Autodesk Inventor part; units mm, degrees
ref_plane "YZ Plane" through (0, 0, 0) normal (1, 0, 0) x (0, 1, 0)
ref_plane "XZ Plane" through (0, 0, 0) normal (0, 1, 0) x (-1, 0, 0)
ref_plane "XY Plane" through (0, 0, 0) normal (0, 0, 1) x (1, 0, 0)
sketch "Sketch1" plane through (0, 0, 0) normal (0, 1, 0) x (-1, 0, 0)
  line L0 (101.6, -38.1) -> (-101.6, -38.1)
  line L1 (-101.6, -38.1) -> (-101.6, 38.1)
  line L2 (-101.6, 38.1) -> (101.6, 38.1)
  line L3 (101.6, 38.1) -> (101.6, -38.1)
  line L4 (101.6, -38.1) -> (-101.6, 38.1) construction
  line L5 (-101.6, -38.1) -> (101.6, 38.1) construction
  point P0 (0, 0)
  dimension "d0" = 203.2
  dimension "d1" = 76.2
extrude "Extrusion1" add sketch "Sketch1" against normal blind 3.175
sketch "Sketch2" plane through (0, 0, 0) normal (0, 1, 0) x (1, 0, 0)
  line L0 (-101.6, 38.1) -> (101.6, 38.1) construction
  line L1 (0, 38.1) -> (0, -38.1) construction
  line L2 (101.6, -38.1) -> (-101.6, -38.1) construction
  point P0 (0, 0)
  point P1 (-63.5, 19.05)
  point P2 (0, 0)
  point P3 (63.5, 19.05)
  dimension "d4" = 19.05
  dimension "d5" = 63.5
hole "Hole1" at (-63.5, 0, -19.05) at (63.5, 0, -19.05) direction (0, -1, 0) diameter 22.225 end through all
fillet "Fillet1" radius 9.525 2 edges at (101.6, -1.5875, 38.1) (-101.6, -1.5875, 38.1)
properties part number "GP2-002" material "Aluminum 6061"
Geometry: final body of the model. Coordinates: model frame, mm. Coordinates: 2 decimals unless noted, no trailing zeros. Order: outer loops, then holes, each group sorted by start corner. A loop starts at its lowest first (then second) coordinate and runs counter-clockwise, first axis right, second up. Notation, with made-up numbers: M -4.5,-2 L 10.5,-2 A28 cw 10.5,22 Z; hole C 75.25,-21 d1. An arc over 180 degrees is marked long. One line per question, with ' | ' between items. Start each with the question number.
Item 1: Cut plane B-B, the plane y = -1.1. Count the separate pieces of the cut face and the enclosed holes in it, then the cut area to 3 significant figures.
Item 2: Ray query, probe 1 along X at (y, z) = (-1.8, -19.05); probe 2 along Z at (x, y) = (63.5, -0.9); probe 3 along X at (y, z) = (-1.8, -13). Return the intervals inside material, ascending. Write a range as [from, to].
Item 3: Cut plane A-A, the plane z = -19.05. Return the cut outline in (x, y) (1 decimal).
Item 4: Cut plane D-D, the plane x = 54.5. Return the cut outline in (y, z) (3 decimals), then the cut area to 3 significant figures.
Item 5: Pin query (flat end, axial travel): pin 1 Ø18 at (x, z) = (-63.5, -19.05) entering from -Y. Return the tip coordinate at first contact, or that it passes through.
Item 6: Draft query along Z for faces 1 (the flat face through (1, 0, 1)), 2 (the cylindrical face through (-74.518, -1.61, -20.497)), 3 (the cylindrical face through (98.88, -1.61, 35.24)). Return one class per face: released by +Z, released by -Z, zero draft, split by the parting line, or undercut.
Item 7: Cut plane C-C, the plane x = -63.5. Return the cut outline in (y, z) (1 decimal), then the cut area to 3 significant figures.
A:
1) separate pieces: 1 | enclosed holes: 2 | area: 14,700 mm2
2) probe 1: x = [-101.6, -74.61], [-52.39, 52.39], [74.61, 101.6] | probe 2: z = [-38.1, -30.16], [-7.94, 38.1] | probe 3: x = [-101.6, -72.82], [-54.18, 54.18], [72.82, 101.6]
3) outline: M -101.6,-3.2 L -74.6,-3.2 L -74.6,0 L -101.6,0 Z; M -52.4,-3.2 L 52.4,-3.2 L 52.4,0 L -52.4,0 Z; M 74.6,-3.2 L 101.6,-3.2 L 101.6,0 L 74.6,0 Z
4) outline: M -3.175,-38.1 L 0,-38.1 L 0,-25.568 L -3.175,-25.568 Z; M -3.175,-12.532 L 0,-12.532 L 0,38.1 L -3.175,38.1 Z | area: 201 mm2
5) pin 1: passes through
6) face 1: zero draft | face 2: undercut | face 3: released by +Z
7) outline: M -3.2,-38.1 L 0,-38.1 L 0,-30.2 L -3.2,-30.2 Z; M -3.2,-7.9 L 0,-7.9 L 0,38.1 L -3.2,38.1 Z | area: 171 mm2
